Geometry: final body of the model. Coordinates: model frame, mm. A direction names the side the tool comes from. Give positions to 0.01 mm unless a question says otherwise; leave off trailing zeros. Order: outer loops, then holes, each group sorted by start corner. A loop starts at its lowest first (then second) coordinate and runs counter-clockwise, first axis right, second up. Notation, with made-up numbers: M -21,-34 L 38,-34 A20 cw 38,-24 Z; hole C -33.75,3 d10. An arc over 180 degrees is marked long. One line per item, written item: value. Start each with the question number.
Autodesk Inventor part; units mm, degrees
ref_plane "YZ Plane" through (0, 0, 0) normal (1, 0, 0) x (0, 1, 0)
ref_plane "XZ Plane" through (0, 0, 0) normal (0, 1, 0) x (-1, 0, 0)
ref_plane "XY Plane" through (0, 0, 0) normal (0, 0, 1) x (1, 0, 0)
sketch "Sketch2" plane through (0, 0, 0) normal (1, 0, 0) x (0, 1, 0)
  line L0 (0, 0) -> (12, 0) construction
  line L1 (12, 0) -> (12, -5)
  line L2 (12, -5) -> (22, -10.7735)
  line L3 (22, -10.7735) -> (22, -13.5)
  line L4 (22, -13.5) -> (0, -13.5)
  line L5 (0, -13.5) -> (0, 0)
  line L6 (12, 0) -> (12, 5)
  line L7 (12, 5) -> (22, 10.7735)
  line L8 (22, 10.7735) -> (22, 13.5)
  line L9 (22, 13.5) -> (0, 13.5)
  line L10 (0, 13.5) -> (0, 0)
  line L11 (0, 0) -> (0, -46.5785) construction
  line L12 (22, -13.5) -> (22, -23.5)
  line L13 (22, -23.5) -> (0, -23.5)
  line L14 (0, -13.5) -> (0, -23.5)
  dimension "d0" = 22
  dimension "d1" = 13.5
  dimension "d2" = 5
  dimension "d3" = 60
  dimension "d4" = 10
  dimension "d16" = 10
revolve "Revolution1" add sketch "Sketch2" angle 360 about axis through (0, 0, 0) along (0, 0, -1)
sketch "Sketch3" plane through (0, 0, 13.5) normal (0, 0, 1) x (1, 0, 0)
  circle A0 centre (0, 0) radius 2.5
  line L0 (-2, 4) -> (2, 4)
  line L1 (2, 4) -> (2, -2.0439)
  line L2 (2, -2.0439) -> (-2, -2.0439)
  line L3 (-2, -2.0439) -> (-2, 4)
  line L4 (-2, 4) -> (2, -2.0439) construction
  line L5 (2, 4) -> (-2, -2.0439) construction
  line L6 (-5.2122, 2.5) -> (6.1572, 2.5) construction
  point P0 (0, 0.9781)
  point P1 (-2, 1.5)
  point P2 (2, 1.5)
  dimension "d6" = 5
  dimension "d7" = 4
  dimension "d9" = 1.5
extrude "Extrusion1" cut sketch "Sketch3" against normal through all contours A0 L1 | L1 A0 L2 L3 | A0 L3 L0 L1 | L3 A0 | A0 L2
sketch "Sketch4" plane through (0, 0, -23.5) normal (0, 0, 1) x (1, 0, 0)
  circle A0 centre (0, -17) radius 3
  arc A1 (-2, 1.5) -> (2, 1.5) centre (0, 0) ccw construction
  line L0 (0, 0) -> (0, -2.5) construction
  line L1 (0, -2.5) -> (0, -17) construction
  line L2 (0, -17) -> (0, -25) construction
  circle A2 centre (0, 0) radius 25 construction
  dimension "d12" = 6
  dimension "d17" = 8
properties part number "Vbelt Drive Pulley"
Q1. Set-up query: faces 5 (the face through (12.52, -1.64, -5.36)), 6 (the face through (-5, 0, -23.5)), 7 (the face through (2, 3, -5)). Return all of +Z, -Z, +X, -X, +Y, -Y with unobstructed straight access to the full face (end or side cutting, diameter ignored); none if empty.
Q2. Section query C-C on z = -19. Return loops of the section in (x, y), and give its area (3 significant figures).
Q3. Ray query, line 1 along X through (y, z) = (0, 0); line 2 along Z through (x, y) = (-9, 13); line 3 along Z through (x, y) = (7, -16). Return the intervals inside material, ascending. Write a range as [from, to].
Q4. Section query D-D on z = -10. Return loops of the section in (x, y).
Q5. Section query B-B on y = 0. Return loops of the section in (x, z).
Q6. Contact query for flat-ended pins moving along their axis: pin 1 (6 mm diameter, centred on y = 17.5, z = 2.5, fed in from -X); pin 2 (1.2 mm diameter, centred on y = 3, z = -12.5, fed in from -X); pin 3 (1.5 mm diameter, centred on y = -7, z = -9, fed in from -X); pin 4 (3 mm diameter, centred on y = 9, z = 5, fed in from +X). Output: stop coordinate, or through.
Q7. Section query A-A on x = 0. Return loops of the section in (y, z), and give its area (3 significant figures).
Q8. Mould query, pull axis X, two halves, no side actions, for faces 1 (the face through (0, 4, -5)), 2 (the face through (-0.1, -2.5, -4.7)), 3 (the face through (-5, 0, 13.5)), 4 (the face through (-21.477, -4.769, -17.226)). Classes: +X half, -X half, draft (parallel to the pull), parting line (faces both ways), or undercut.
Results below:
1. face 5: none
1. face 6: -Z, +X, -X, +Y, -Y
1. face 7: +Z, -Z
2. outline: C 0,0 d44; hole M -2,1.5 A2.5 ccw long 2,1.5 L 2,4 L -2,4 Z
2. area: 1,490 mm2
3. line 1: [-12, -2.5], [2.5, 12]
3. line 2: [-23.5, -7.2], [7.2, 13.5]
3. line 3: [-23.5, -8.15], [8.15, 13.5]
4. outline: C 0,0 d41.32; hole M -2,1.5 A2.5 ccw long 2,1.5 L 2,4 L -2,4 Z
5. outline: M -22,-23.5 L -2.5,-23.5 L -2.5,13.5 L -22,13.5 L -22,10.77 L -12,5 L -12,-5 L -22,-10.77 Z; M 2.5,-23.5 L 22,-23.5 L 22,-10.77 L 12,-5 L 12,5 L 22,10.77 L 22,13.5 L 2.5,13.5 Z
6. pin 1: through
6. pin 2: x = -21.87
6. pin 3: x = -19
6. pin 4: x = 11.69
7. outline: M -22,-23.5 L -2.5,-23.5 L -2.5,13.5 L -22,13.5 L -22,10.77 L -12,5 L -12,-5 L -22,-10.77 Z; M 4,-23.5 L 22,-23.5 L 22,-10.77 L 12,-5 L 12,5 L 22,10.77 L 22,13.5 L 4,13.5 Z
7. area: 1,070 mm2
8. face 1: undercut
8. face 2: undercut
8. face 3: draft
8. face 4: parting line
